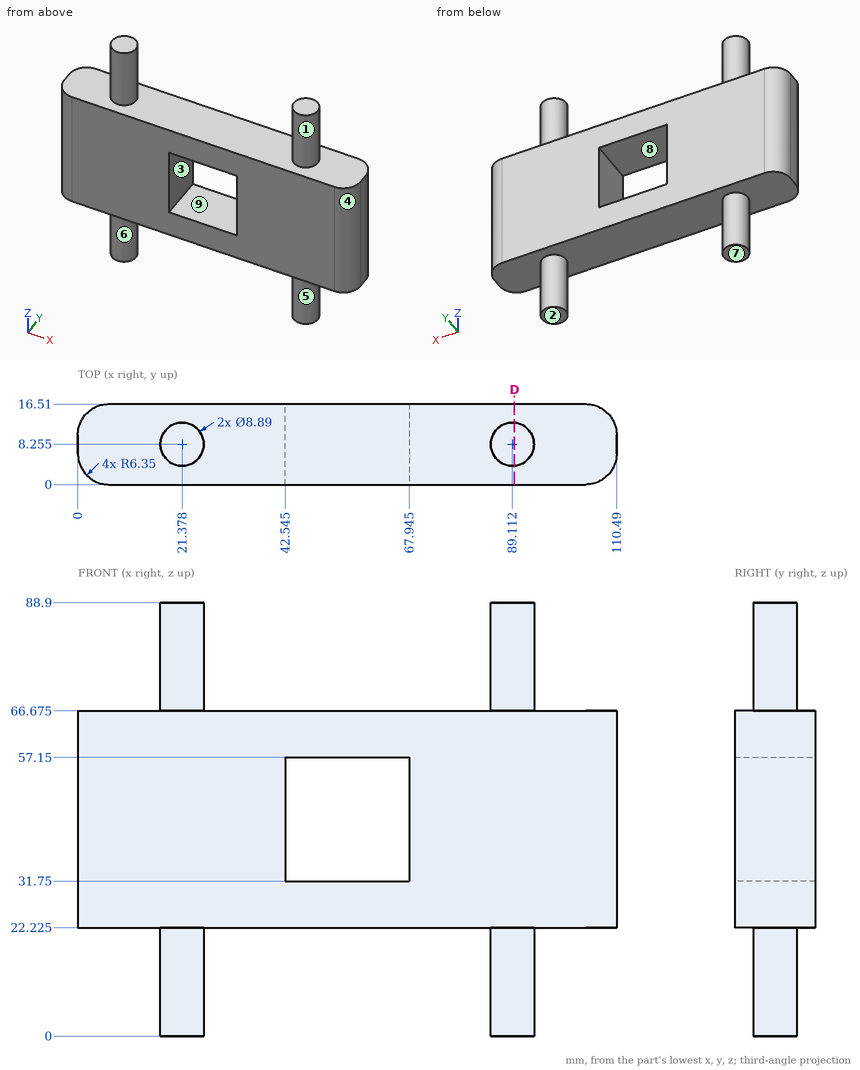
Part print with two shaded views. Sizes in mm from the minimum x, y, z corner. A direction names the side the tool comes from. Round coordinates to 2 decimals unless told otherwise and drop trailing zeros. Write each loop counter-clockwise with the first axis right and the second up, starting at its lowest first coordinate (ties: lowest second). Pieces come first, ordered by that corner, then holes. Notation, with made-up numbers: M 28.5,40 L 60.5,40 A32 ccw 60.5,76 Z; hole C -24,80 d5. An arc over 180 degrees is marked long. Put each result on its own line as item: value. Start each with the question number.
1) Drill centre lines: probe 1 along X at (y, z) = (10, 32.5) (1 decimal); probe 2 along Z at (x, y) = (77, 14.25) (1 decimal); probe 3 along X at (y, z) = (7.75, 85) (1 decimal). Where is each one in solid material? Low to high. Write a range as [from, to].
2) 3-axis set-ups, long thin cutter, end or side, ignore diameter. For the marked faces 1, 2, 3, 4 and 5: which of +Z, -Z, +X, -X, +Y, -Y reach the whole face in a straight line?
3) Pull direction Z, two halves, no side cores. Call the marked faces 6, 7, 8 and 9: pulls with the +Z half, pulls with the -Z half, needs draft (parallel to the pull), parting line crosses it, or undercut.
4) Saw through at D-D, the plane x = 89.5. Write the cut outline in (y, z) (1 decimal).
5) Pin check, flat tips, straight feed: pin 1 Ø8.5 at (x, y) = (50, 9) entering from -Z (3 decimals); pin 2 Ø1.5 at (y, z) = (2, 23) entering from -X; pin 3 Ø5 at (x, y) = (52.5, 11.5) entering from +Z (3 decimals). Stop position of each tip, or through.
Resolved:
1. probe 1: [0, 42.5], [67.9, 110.5]
1. probe 2: [22.2, 66.7]
1. probe 3: [17, 25.8], [84.7, 93.5]
2. face 1: +Z
2. face 2: -Z, +X, -X, +Y, -Y
2. face 3: +Y, -Y
2. face 4: +Z, -Z, +X, -Y
2. face 5: -Z
3. face 6: needs draft
3. face 7: pulls with the -Z half
3. face 8: undercut
3. face 9: undercut
4. outline: M 0,22.2 L 3.8,22.2 L 3.8,0 L 12.7,0 L 12.7,22.2 L 16.5,22.2 L 16.5,66.7 L 12.7,66.7 L 12.7,88.9 L 3.8,88.9 L 3.8,66.7 L 0,66.7 Z
5. pin 1: z = 22.225
5. pin 2: x = 1.12
5. pin 3: z = 66.675
